For this review, take the finished solid that the model builds, in its own axes (mm). Face numbers are marked on the shaded views. A direction names the side the tool comes from. Coordinates: 2 decimals unless noted, no trailing zeros. Write each loop counter-clockwise with the first axis right and the second up, starting at its lowest first coordinate (ties: lowest second). Pieces come first, ordered by that corner, then holes.
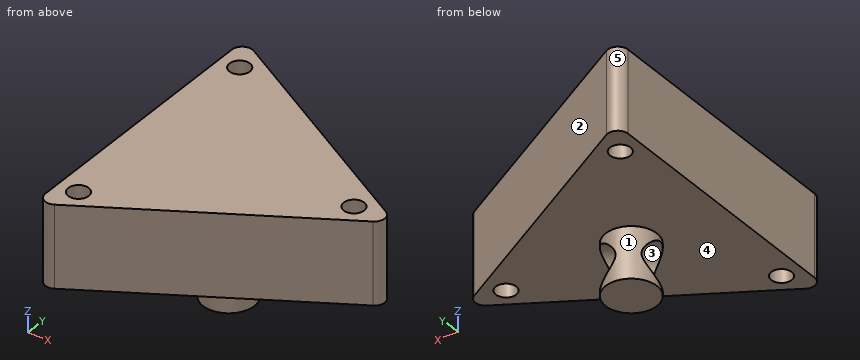
```python
from build123d import *

# Parameters (mm, degrees)
Y_KSEKLIK_EKSTR_ZYON1_DEPTH = 16
IZIM2_W                     = 5
IZIM2_H                     = 10
F_4_0_4_AP_DELIK1_D         = 4
M8_BO_LUKLU_DELIK1_D        = 8.55
M8_BO_LUKLU_DELIK1_DEPTH    = 34.043716459


with BuildPart() as part:
    # Çizim1 → Yükseklik-Ekstrüzyon1 (new body)
    with BuildSketch(Plane(origin=(0, 0, 0), x_dir=(-1, 0, 0), z_dir=(0, 0, -1))):
        with BuildLine():
            Line((24.144741863, 27.209326424), (-19.863531155, 1.730852571))
            ThreePointArc((-19.863531155, 1.730852571), (-20.861458614, 0), (-19.863531155, -1.730852571))
            Line((-19.863531155, -1.730852571), (24.144741863, -27.209326424))
            ThreePointArc((24.144741863, -27.209326424), (26.145777596, -27.211122848), (27.146814404, -25.478473853))
            Line((27.146814404, -25.478473853), (27.146814404, 25.478473853))
            ThreePointArc((27.146814404, 25.478473853), (26.145777596, 27.211122848), (24.144741863, 27.209326424))
        make_face()
    extrude(amount=-Y_KSEKLIK_EKSTR_ZYON1_DEPTH)

    # Çizim2 → Döndür1 (revolve)
    with BuildSketch(Plane(origin=(0, -0.521526147, 0), x_dir=(1, 0, 0), z_dir=(0, 1, 0))):
        with Locations((-6.693456416, 5)):
            Rectangle(IZIM2_W, IZIM2_H)
    revolve(axis=Axis((-9.193456416, -0.521526147, -10), (0, 0, 1)))

    # Ø4.0 (4) Çap Delik1 (through all)
    with Locations(Plane(origin=(0, 0, 0), x_dir=(-1, 0, 0), z_dir=(0, 0, -1))):
        with Locations((23.146814404, -22.009579284), (-14.869731632, 0), (23.146814404, 22.009579284)):
            Hole(F_4_0_4_AP_DELIK1_D / 2)

    # M8 Boşluklu Delik1
    with Locations(Plane(origin=(-2.784563035, -1.612115441, 0), x_dir=(0, 0, -1), z_dir=(0.8654262854811261, 0.501036270541705, 0))):
        with Locations((5, 4.433526161)):
            Hole(M8_BO_LUKLU_DELIK1_D / 2, depth=M8_BO_LUKLU_DELIK1_DEPTH)


solid = part.part
```
Q1. For probe 1 along Y at (x, z) = (-24.5, 8.25); probe 2 along Z at (x, y) = (-15, -4); probe 3 along X at (y, z) = (23.5, 10), list the stretches that pass through material, from the lowest coordinate up.
Ans:
probe 1: y = -27.37 to -23.48, -20.54 to 20.54, 23.48 to 27.37
probe 2: z = 0 to 16
probe 3: x = -27.15 to -24.48, -21.81 to -17.74
Q2. Tool access review of the marked faces 1 and 2: name each direction out of +Z, -Z, +X, -X, +Y, -Y from which nothing blocks a thin tool from reaching the whole face with its end or side.
Ans:
face 1: -Z
face 2: +Z, -Z, +X, +Y
Q3. Add section D-D (z = -7.25). State the section outline as (x, y) points, then the cut area to 3 significant figures.
Ans:
outline: (-13.85, 1.31) - (-8.46, 4.42) arc R5 ccw to start; (-10.72, -5.28) arc R5 ccw to (-4.3, -1.57) - close
area: 13.0 mm2
Q4. Add section A-A (z = 2). State the section outline as (x, y) points.
Ans:
outline: (-27.15, -25.48) arc R2 ccw to (-24.14, -27.21) - (19.86, -1.73) arc R2 ccw to (19.86, 1.73) - (-24.14, 27.21) arc R2 ccw to (-27.15, 25.48) - close; hole circle Ø4 at (-23.15, -22.01); hole circle Ø4 at (-23.15, 22.01); hole circle Ø4 at (14.87, 0)
Q5. Draft analysis for pull direction Z (two halves, no side actions). For the marked faces 3, 4 and 5, state which applies: +Z half, -Z half, draft (parallel to the pull), parting line (faces both ways), or undercut.
Ans:
face 3: undercut
face 4: -Z half
face 5: draft
Q6. Add section B-B (x = 5.5). State the section outline as (y, z) points, then the cut area to 3 significant figures.
Ans:
outline: (-10.05, 0) - (10.05, 0) - (10.05, 16) - (-10.05, 16) - close
area: 321 mm2
Q7. Add section C-C (y = -19). State the section outline as (x, z) points (3 decimals), then the cut area to 3 significant figures.
Ans:
outline: (-27.147, 0) - (-9.965, 0) - (-9.965, 16) - (-27.147, 16) - close
area: 275 mm2
Q8. Clearance check with flat-ended pins moving along their axes: pin 1 Ø1.5 at (x, z) = (-13, -6.5) entering from -Y; pin 2 Ø10 at (x, z) = (-1.5, 7.5) entering from +Y; pin 3 Ø4.5 at (x, y) = (-23.15, 22.01) entering from -Z. State where each tip first meets the part, or that it passes through.
Ans:
pin 1: stops at y = 1.64
pin 2: stops at y = 16.99
pin 3: stops at z = 0
